Check sheet for the drawn part. Datum: minimum x, y, z corner. Units: mm. Give positions to 0.01 mm unless a question says otherwise; leave off trailing zeros. Order: outer loops, then holes, each group sorted by start corner. A loop starts at its lowest first (then second) coordinate and runs counter-clockwise, first axis right, second up. Notation, with made-up numbers: (-37.5, 7.5) -> (-4.5, 7.5) arc R10 cw to (-4.5, 11.5) -> close; hole circle Ø10 at (-21, 34.25). An arc over 180 degrees is marked (long way). Answer in a Markdown table with one row per item. Add a question column.
(1) Cross-section at A-A (y = 40). Record the cut outline in (x, z), then the cut area to 3 significant figures.
(2) Thickness scan on L1, parallel to Y at x = 17, z = 3.7; L2, parallel to Y at x = 3, z = 2.2; L3, parallel to X at y = 58, z = 3.4. Record the ranges inside material, lowest first. Write a range as [from, to].
(3) Cross-section at C-C (x = 17). Record the cut outline in (y, z).
(4) Cross-section at D-D (z = 4.8). Record the cut outline in (x, y), then the cut area to 3 significant figures.
(5) Release check for a two-part mould opening along X. For the marked faces 1, 2, 3 and 4 record: released by +X, released by -X, zero draft, split by the parting line, or undercut.
(6) Cross-section at B-B (x = 3). Record the cut outline in (y, z), then the cut area to 3 significant figures.
(7) Go/stop test with a flat-tipped pin: pin 1 (15 mm diameter, centred on x = 21.5, y = 16.5, fed in from -Z). Record where the tip stops, or that it passes through.
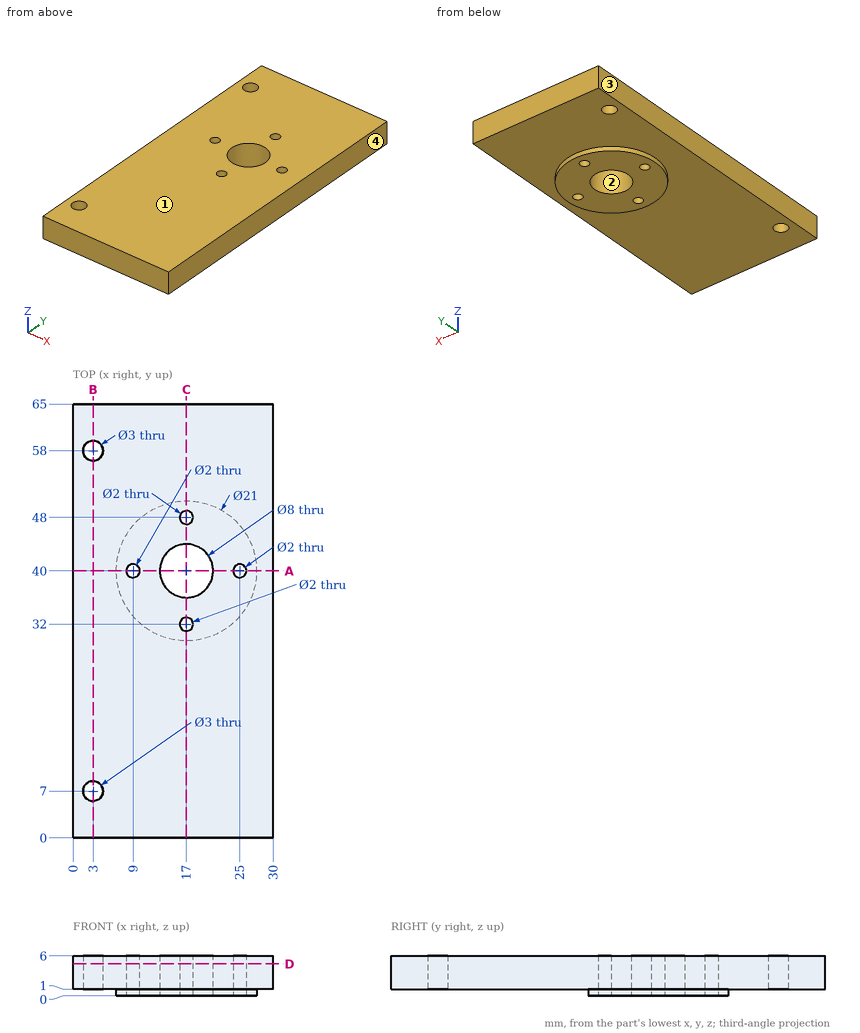
Answer below:
| question | item | result |
|---|---|---|
| 1 | outline | (0, 1) -> (6.5, 1) -> (6.5, 0) -> (8, 0) -> (8, 6) -> (0, 6) -> close; (10, 0) -> (13, 0) -> (13, 6) -> (10, 6) -> close; (21, 0) -> (24, 0) -> (24, 6) -> (21, 6) -> close; (26, 0) -> (27.5, 0) -> (27.5, 1) -> (30, 1) -> (30, 6) -> (26, 6) -> close |
| 1 | area | 99.0 mm² |
| 2 | L1 | y = [0, 31], [33, 36], [44, 47], [49, 65] |
| 2 | L2 | y = [0, 5.5], [8.5, 56.5], [59.5, 65] |
| 2 | L3 | x = [0, 1.5], [4.5, 30] |
| 3 | outline | (0, 1) -> (29.5, 1) -> (29.5, 0) -> (31, 0) -> (31, 6) -> (0, 6) -> close; (33, 0) -> (36, 0) -> (36, 6) -> (33, 6) -> close; (44, 0) -> (47, 0) -> (47, 6) -> (44, 6) -> close; (49, 0) -> (50.5, 0) -> (50.5, 1) -> (65, 1) -> (65, 6) -> (49, 6) -> close |
| 4 | outline | (0, 0) -> (30, 0) -> (30, 65) -> (0, 65) -> close; hole circle Ø3 at (3, 7); hole circle Ø3 at (3, 58); hole circle Ø2 at (9, 40); hole circle Ø8 at (17, 40); hole circle Ø2 at (17, 32); hole circle Ø2 at (17, 48); hole circle Ø2 at (25, 40) |
| 4 | area | 1,870 mm² |
| 5 | face 1 | zero draft |
| 5 | face 2 | undercut |
| 5 | face 3 | released by -X |
| 5 | face 4 | released by +X |
| 6 | outline | (0, 1) -> (5.5, 1) -> (5.5, 6) -> (0, 6) -> close; (8.5, 1) -> (56.5, 1) -> (56.5, 6) -> (8.5, 6) -> close; (59.5, 1) -> (65, 1) -> (65, 6) -> (59.5, 6) -> close |
| 6 | area | 295 mm² |
| 7 | pin 1 | stops at z = 1 |
